CAD build for the part. Positions are in the model's coordinates, mm. Face numbers are marked on the shaded views. A direction names the side the tool comes from. Give positions to 0.01 mm unless a question says otherwise; leave off trailing zeros. Write each loop counter-clockwise with the first axis right and the second up, starting at its lowest first coordinate (ties: lowest second). Pieces come first, ordered by that corner, then holes. Notation, with made-up numbers: (-37, 67.25) -> (1, 67.25) arc R31 ccw to (1, 91.25) -> close; hole circle Ø11 at (-21.5, 57.5). An arc over 180 degrees is marked (long way). Answer as a JSON object with one key per item and string values.
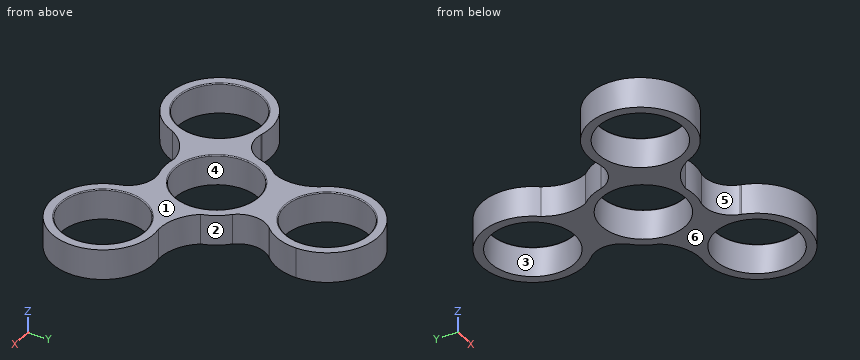
```python
from build123d import *

# Parameters (mm, degrees)
F0_R     = 11.1
F1_DEPTH = 8
F2_R     = 0.25


# Not quite as in the source:
# - a feature of the source that left no trace in its solid (it failed there, or was rolled back) is left out


with BuildPart() as f1:
    # F0 (on Top) → F1 (new body)
    with BuildSketch(Plane.XY):
        with BuildLine():
            ThreePointArc((3.859865491, -12.9364383967), (10.8249291944, -8.0666540731), (13.5, 0))
            ThreePointArc((13.5, 0), (13.3707834369, 1.8633706782), (12.9856073653, 3.691070489))
            ThreePointArc((12.9856073653, 3.691070489), (11.5424684167, 7.0015300363), (9.2733515405, 9.8109607688))
            ThreePointArc((9.2733515405, 9.8109607688), (-0.2922686684, 13.4968358894), (-9.6893644933, 9.4003306174))
            ThreePointArc((-9.6893644933, 9.4003306174), (-11.8347370851, 6.4953058532), (-13.1332170315, 3.1254776279))
            ThreePointArc((-13.1332170315, 3.1254776279), (-11.5424684167, -7.0015300363), (-3.296242872, -13.0914011064))
            ThreePointArc((-3.296242872, -13.0914011064), (0.2922686684, -13.4968358894), (3.859865491, -12.9364383967))
        make_face()
        Circle(F0_R, mode=Mode.SUBTRACT)
        with BuildLine():
            ThreePointArc((12.9856073653, 3.691070489), (13.3707834369, 1.8633706782), (13.5, 0))
            ThreePointArc((13.5, 0), (10.8249291944, -8.0666540731), (3.859865491, -12.9364383967))
            ThreePointArc((3.859865491, -12.9364383967), (8.9875948966, -13.8732661585), (12.1902212779, -17.985982946))
            ThreePointArc((12.1902212779, -17.985982946), (13.9354582524, -7.2213929241), (23.0659975588, -1.2585494405))
            ThreePointArc((23.0659975588, -1.2585494405), (17.4140534965, -0.0296267076), (12.9856073653, 3.691070489))
        make_face()
        with BuildLine():
            ThreePointArc((-9.6893644933, 9.4003306174), (-0.2922686684, 13.4968358894), (9.2733515405, 9.8109607688))
            ThreePointArc((9.2733515405, 9.8109607688), (7.5208034785, 14.7201185786), (9.4812075043, 19.5500327774))
            ThreePointArc((9.4812075043, 19.5500327774), (-0.7138194032, 15.679157322), (-10.443062992, 20.6050145698))
            ThreePointArc((-10.443062992, 20.6050145698), (-8.6813692668, 15.0958260647), (-9.6893644933, 9.4003306174))
        make_face()
        with BuildLine():
            ThreePointArc((38.7535366191, -14.580136165), (33.9919066812, -4.2898063036), (23.0659975588, -1.2585494405))
            ThreePointArc((23.0659975588, -1.2585494405), (13.9354582524, -7.2213929241), (12.1902212779, -17.985982946))
            ThreePointArc((12.1902212779, -17.985982946), (12.2464624781, -18.1789066882), (12.297383992, -18.3733022703))
            ThreePointArc((12.297383992, -18.3733022703), (27.1695141155, -27.9434826858), (38.7535366191, -14.580136165))
        make_face()
        with Locations((25.2535366191, -14.580136165)):
            Circle(F0_R, mode=Mode.SUBTRACT)
        with BuildLine():
            ThreePointArc((-12.6229345668, -19.3464651293), (-8.7326842297, -15.066199357), (-3.296242872, -13.0914011064))
            ThreePointArc((-3.296242872, -13.0914011064), (-11.5424684167, -7.0015300363), (-13.1332170315, 3.1254776279))
            ThreePointArc((-13.1332170315, 3.1254776279), (-16.508398375, -0.8468524201), (-21.6714287822, -1.5640498314))
            ThreePointArc((-21.6714287822, -1.5640498314), (-14.5155559943, -6.3980965598), (-11.7535366191, -14.580136165))
            ThreePointArc((-11.7535366191, -14.580136165), (-11.9726645147, -17.0026216958), (-12.6229345668, -19.3464651293))
        make_face()
        with BuildLine():
            ThreePointArc((12.297383992, -18.3733022703), (12.2464624781, -18.1789066882), (12.1902212779, -17.985982946))
            ThreePointArc((12.1902212779, -17.985982946), (12.24236133, -18.1800413854), (12.297383992, -18.3733022703))
        make_face()
        with BuildLine():
            ThreePointArc((9.7630545215, 19.8364980723), (9.620163766, 19.6952009566), (9.4812075043, 19.5500327774))
            ThreePointArc((9.4812075043, 19.5500327774), (9.6231970167, 19.6922166068), (9.7630545215, 19.8364980723))
        make_face()
        with BuildLine():
            ThreePointArc((-10.443062992, 20.6050145698), (-0.7138194032, 15.679157322), (9.4812075043, 19.5500327774))
            ThreePointArc((9.4812075043, 19.5500327774), (9.620163766, 19.6952009566), (9.7630545215, 19.8364980723))
            ThreePointArc((9.7630545215, 19.8364980723), (12.5309863148, 24.1378842547), (13.5, 29.16027233))
            ThreePointArc((13.5, 29.16027233), (-4.5425020422, 41.8730877223), (-10.443062992, 20.6050145698))
        make_face()
        with Locations((0, 29.16027233)):
            Circle(F0_R, mode=Mode.SUBTRACT)
        with BuildLine():
            ThreePointArc((-22.0604385135, -1.463195802), (-37.1929755561, -20.8809137257), (-12.6229345668, -19.3464651293))
            ThreePointArc((-12.6229345668, -19.3464651293), (-11.9726645147, -17.0026216958), (-11.7535366191, -14.580136165))
            ThreePointArc((-11.7535366191, -14.580136165), (-14.5155559943, -6.3980965598), (-21.6714287822, -1.5640498314))
            ThreePointArc((-21.6714287822, -1.5640498314), (-21.8666262441, -1.5162942684), (-22.0604385135, -1.463195802))
        make_face()
        with Locations((-25.2535366191, -14.580136165)):
            Circle(F0_R, mode=Mode.SUBTRACT)
        with BuildLine():
            ThreePointArc((-22.0604385135, -1.463195802), (-21.8666262441, -1.5162942684), (-21.6714287822, -1.5640498314))
            ThreePointArc((-21.6714287822, -1.5640498314), (-21.8655583466, -1.5121752213), (-22.0604385135, -1.463195802))
        make_face()
    extrude(amount=F1_DEPTH)

    # F2
    f2_edges = [f1.edges().sort_by_distance(p)[0] for p in [
        (-11.1, 29.160272, 8),
        (-36.353537, -14.580136, 8),
        (14.153537, -14.580136, 8),
        (-11.1, 0, 8),
    ]]
    fillet(f2_edges, radius=F2_R)


solid = f1.part
```
1) Slice it at A-A (x = 0). List the corners of the cut face in (y, z), then the cut area to 3 significant figures.
Model answer:
{"outline": "(-13.5, 0) -> (-11.1, 0) -> (-11.1, 7.75) arc R0.25 ccw to (-11.35, 8) -> (-13.5, 8) -> close; (11.1, 0) -> (18.06, 0) -> (18.06, 7.75) arc R0.25 ccw to (17.81, 8) -> (11.35, 8) arc R0.25 ccw to (11.1, 7.75) -> close; (40.26, 0) -> (42.66, 0) -> (42.66, 8) -> (40.51, 8) arc R0.25 ccw to (40.26, 7.75) -> close", "area": "94.0 mm2"}
2) Slice it at B-B (y = 0). List the corners of the cut face in (x, z).
Model answer:
{"outline": "(-15.28, 0) -> (-11.1, 0) -> (-11.1, 7.75) arc R0.25 ccw to (-11.35, 8) -> (-15.28, 8) -> close; (11.1, 0) -> (17.35, 0) -> (17.35, 8) -> (11.35, 8) arc R0.25 ccw to (11.1, 7.75) -> close"}
3) 3-axis set-ups, long thin cutter, end or side, ignore diameter. For the marked faces 1 and 2: which of +Z, -Z, +X, -X, +Y, -Y reach the whole face in a straight line?
Model answer:
{"face 1": "+Z, +X, -X, +Y, -Y", "face 2": "+Z, -Z, +X"}
4) Wall check: probe 1 along X at (y, z) = (-24, 1.25); probe 2 along Y at (x, z) = (0, 4.75); probe 3 along X at (y, z) = (-4.5, 7.5). Give the ranges that are in metal, low to high.
Model answer:
{"probe 1": "x = -34.92 to -31.13, -19.38 to -15.58, 15.58 to 19.38, 31.13 to 34.92", "probe 2": "y = -13.5 to -11.1, 11.1 to 18.06, 40.26 to 42.66", "probe 3": "x = -34.23 to -29.9, -20.61 to -10.15, 10.15 to 20.61, 29.9 to 34.23"}
5) Slice it at C-C (z = 5.5). List the corners of the cut face in (x, y).
Model answer:
{"outline": "(-21.67, -1.56) arc R13.5 ccw (long way) to (-12.62, -19.35) arc R12.05 cw to (-3.3, -13.09) arc R13.5 ccw to (3.86, -12.94) arc R7.32 cw to (12.19, -17.99) arc R13.5 ccw (long way) to (23.07, -1.26) arc R12.05 cw to (12.99, 3.69) arc R13.5 ccw to (9.27, 9.81) arc R7.32 cw to (9.48, 19.55) arc R13.5 ccw (long way) to (-10.44, 20.61) arc R12.05 cw to (-9.69, 9.4) arc R13.5 ccw to (-13.13, 3.13) arc R7.32 cw to start; hole circle Ø22.2 at (-25.25, -14.58); hole circle Ø22.2 at (0, 0); hole circle Ø22.2 at (0, 29.16); hole circle Ø22.2 at (25.25, -14.58)"}
6) Pin check, flat tips, straight feed: pin 1 (2 mm diameter, centred on x = 15.5, z = 2, fed in from -Y); pin 2 (2 mm diameter, centred on y = -5.5, z = 5, fed in from +X). Stop position of each tip, or through.
Model answer:
{"pin 1": "stops at y = -24.86", "pin 2": "stops at x = 36.07"}
7) Mould opens along Y. For the marked faces 3, 4, 5 and 6 say: released by +Y, released by -Y, zero draft, split by the parting line, or undercut.
Model answer:
{"face 3": "undercut", "face 4": "undercut", "face 5": "released by -Y", "face 6": "zero draft"}
